Input: part model. Units: mm. Frame: model coordinates. Coordinates: 2 decimals unless noted, no trailing zeros. Write each loop counter-clockwise with the first axis right and the second up, starting at its lowest first coordinate (ties: lowest second). Pieces come first, ordered by that corner, then holes. Notation, with made-up numbers: M 29.5,77 L 56.5,77 A20 ccw 56.5,91 Z; hole C -37,-3 d7. An arc over 180 degrees is marked long. Answer as a JSON object with one key per item and string values. Group by question number.
from build123d import *

# Parameters (mm, degrees)
CROQUIS1_W              = 200
CROQUIS1_H              = 100
SALIENTE_EXTRUIR1_DEPTH = 20
CROQUIS2_R              = 7
CORTAR_EXTRUIR1_DEPTH   = 9
CROQUIS3_R              = 4.25
CORTAR_EXTRUIR2_DEPTH   = 113.343224095


with BuildPart() as part:
    # Croquis1 → Saliente-Extruir1 (new body)
    with BuildSketch(Plane(origin=(0, 0, 0), x_dir=(1, 0, 0), z_dir=(0, 1, 0))):
        Rectangle(CROQUIS1_W, CROQUIS1_H)
    extrude(amount=SALIENTE_EXTRUIR1_DEPTH)

    # Croquis2 → Cortar-Extruir1 (cut)
    with BuildSketch(Plane.XZ):
        with Locations(Location((-18, 18, 0), (0, 0, 270))):
            Circle(CROQUIS2_R)
        with Locations(Location((-18, -18, 0), (0, 0, 270))):
            Circle(CROQUIS2_R)
        with Locations(Location((18, 18, 0), (0, 0, 270))):
            Circle(CROQUIS2_R)
        with Locations(Location((18, -18, 0), (0, 0, 270))):
            Circle(CROQUIS2_R)
    extrude(amount=-CORTAR_EXTRUIR1_DEPTH, mode=Mode.SUBTRACT)

    # Croquis3 → Cortar-Extruir2 (cut, through all)
    with BuildSketch(Plane.XZ.offset(-9)):
        with Locations(Location((-18, 18, 0), (0, 0, 270))):
            Circle(CROQUIS3_R)
        with Locations(Location((18, 18, 0), (0, 0, 270))):
            Circle(CROQUIS3_R)
        with Locations(Location((18, -18, 0), (0, 0, 270))):
            Circle(CROQUIS3_R)
        with Locations(Location((-18, -18, 0), (0, 0, 270))):
            Circle(CROQUIS3_R)
    extrude(amount=-CORTAR_EXTRUIR2_DEPTH, mode=Mode.SUBTRACT)


solid = part.part
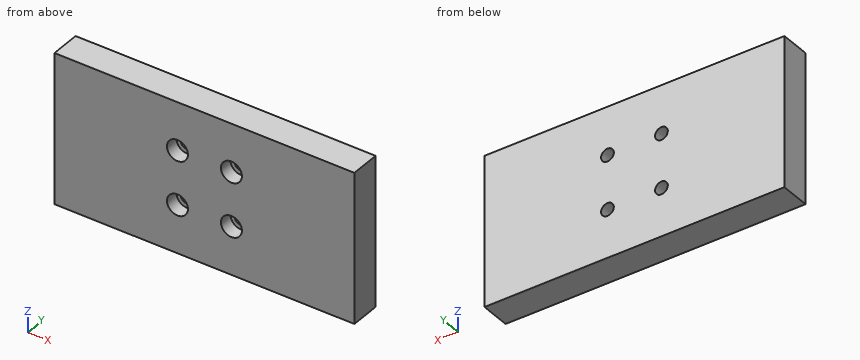
Q1. Section A-A, the plane z = -18. Return the cut outline in (x, y).
Q2. Section C-C, the plane x = -18. Return the cut outline in (y, z).
Q3. Line query: line 1 (X direction, y = 3, z = 18); line 2 (X direction, y = 11.75, z = -18); line 3 (Z direction, x = 20, y = 10). Output: solid intervals per line, ascending. Write a range as from..to.
Q4. Section B-B, the plane y = 7. Return the cut outline in (x, z).
Q5. Pin query (flat end, axial travel): pin 1 Ø10 at (x, z) = (18, 18) entering from -Y. Return the tip coordinate at first contact, or that it passes through.
Filled in:
{
 "1": {"outline": "M -100,0 L -25,0 L -25,9 L -22.25,9 L -22.25,20 L -100,20 Z; M -13.75,9 L -11,9 L -11,0 L 11,0 L 11,9 L 13.75,9 L 13.75,20 L -13.75,20 Z; M 22.25,9 L 25,9 L 25,0 L 100,0 L 100,20 L 22.25,20 Z"},
 "2": {"outline": "M 0,-50 L 20,-50 L 20,-22.25 L 9,-22.25 L 9,-25 L 0,-25 Z; M 0,-11 L 9,-11 L 9,-13.75 L 20,-13.75 L 20,13.75 L 9,13.75 L 9,11 L 0,11 Z; M 0,25 L 9,25 L 9,22.25 L 20,22.25 L 20,50 L 0,50 Z"},
 "3": {"line 1": "-100..-25, -11..11, 25..100", "line 2": "-100..-22.25, -13.75..13.75, 22.25..100", "line 3": "-50..-21.75, -14.25..14.25, 21.75..50"},
 "4": {"outline": "M -100,-50 L 100,-50 L 100,50 L -100,50 Z; hole C -18,-18 d14; hole C -18,18 d14; hole C 18,-18 d14; hole C 18,18 d14"},
 "5": {"pin 1": "y = 9"}
}
